Verification items for this drawing (mm, ordinates from the low corner). A direction names the side the tool comes from. Give positions to 0.01 mm unless a question says otherwise; leave off trailing zeros. Loops run counter-clockwise (first coordinate to the right, second up) from the corner with the lowest first, then second, coordinate; pieces in that order, holes last. Notation, with made-up numbers: M 61.25,58 L 111.25,58 A33 ccw 111.25,94 Z; hole C 10.25,83.5 d2. An arc over 180 degrees is marked long. Use one line per item in the form item = value.
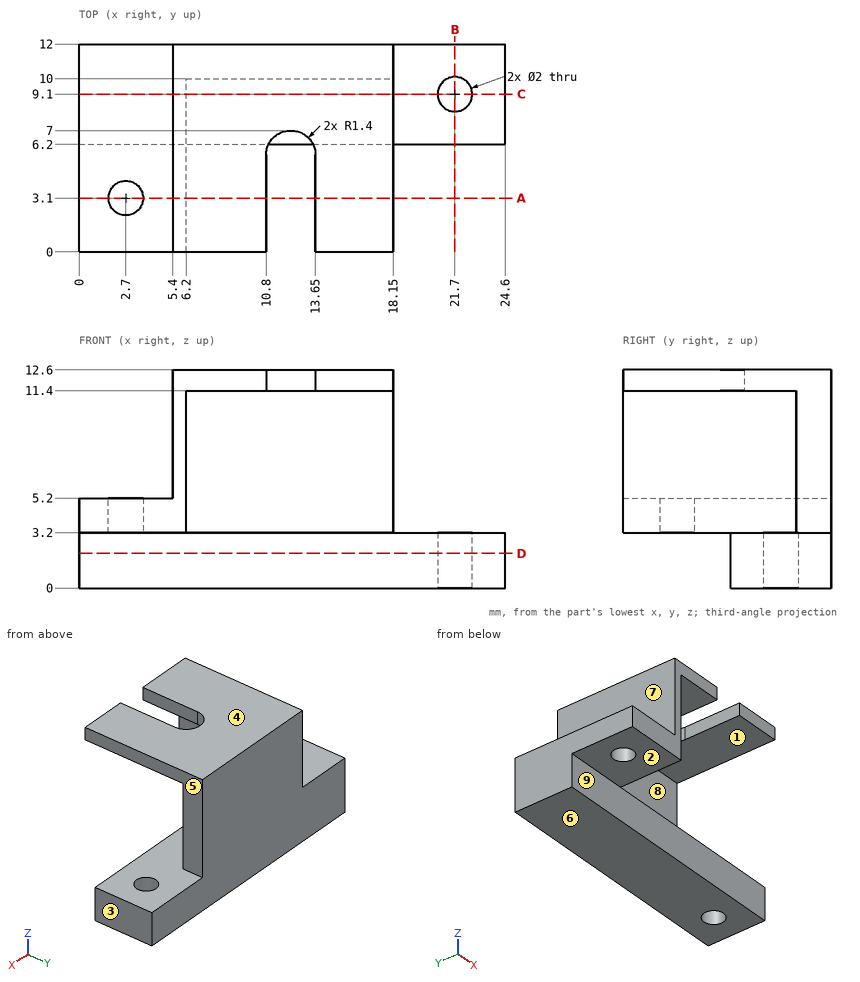
1) Section check A-A (y = 3.1). Record the cut outline in (x, z).
Evaluation:
outline = M 0,3.2 L 1.7,3.2 L 1.7,5.2 L 0,5.2 Z; M 3.7,3.2 L 6.2,3.2 L 6.2,11.4 L 10.8,11.4 L 10.8,12.6 L 5.4,12.6 L 5.4,5.2 L 3.7,5.2 Z; M 13.65,11.4 L 18.15,11.4 L 18.15,12.6 L 13.65,12.6 Z
2) Section check D-D (z = 2). Record the cut outline in (x, y), then the cut area to 3 significant figures.
Evaluation:
outline = M 0,6.2 L 24.6,6.2 L 24.6,12 L 0,12 Z; hole C 21.7,9.1 d2
area = 140 mm^2
3) Scan lines: line 1 (Y direction, x = 2.7, z = 4.05); line 2 (Y direction, x = 21.7, z = 2.1); line 3 (Z direction, x = 9.5, y = 8). Record each from-to range of solid material in increasing order.
Evaluation:
line_1 = 0 to 2.1, 4.1 to 12
line_2 = 6.2 to 8.1, 10.1 to 12
line_3 = 0 to 3.2, 11.4 to 12.6
4) Depth check by flat-ended pin: pin 1 Ø6 at (x, z) = (17, 2.5) entering from -Y; pin 2 Ø1.3 at (y, z) = (3, 12) entering from +X; pin 3 Ø2.5 at (x, y) = (2.7, 3.1) entering from -Z; pin 4 Ø1.8 at (x, y) = (21.7, 9.1) entering from -Z. Enter the tip coordinate at first touch or a pass-through.
Evaluation:
pin_1 = 6.2
pin_2 = 18.15
pin_3 = 3.2
pin_4 = through
5) Set-up check for the marked faces 5, 6, 7, 8 and 9: record each of +Z, -Z, +X, -X, +Y, -Y from which the full face is reachable in a straight line by a thin tool's end or side.
Evaluation:
face_5 = +Z, +X, +Y, -Y
face_6 = -Z, +X, -X, +Y, -Y
face_7 = +Z, -X, +Y, -Y
face_8 = +X, -Y
face_9 = -Z, +X, -X, -Y
6) Section check B-B (x = 21.7). Record the cut outline in (y, z).
Evaluation:
outline = M 6.2,0 L 8.1,0 L 8.1,3.2 L 6.2,3.2 Z; M 10.1,0 L 12,0 L 12,3.2 L 10.1,3.2 Z
7) Release check for a two-part mould opening along Z. For the marked faces 1, 2, 3 and 4 record: pulls with the +Z half, pulls with the -Z half, needs draft (parallel to the pull), parting line crosses it, or undercut.
Evaluation:
face_1 = undercut
face_2 = pulls with the -Z half
face_3 = needs draft
face_4 = pulls with the +Z half
8) Section check C-C (y = 9.1). Record the cut outline in (x, z), then the cut area to 3 significant figures.
Evaluation:
outline = M 0,0 L 20.7,0 L 20.7,3.2 L 6.2,3.2 L 6.2,11.4 L 18.15,11.4 L 18.15,12.6 L 5.4,12.6 L 5.4,5.2 L 0,5.2 Z; M 22.7,0 L 24.6,0 L 24.6,3.2 L 22.7,3.2 Z
area = 105 mm^2
